Design review of the part built by this model. Coordinates are the model's own, in mm. Round coordinates to 2 decimals unless told otherwise and drop trailing zeros. Order: outer loops, then holes, each group sorted by start corner. A loop starts at its lowest first (then second) coordinate and runs counter-clockwise, first axis right, second up. Notation, with made-up numbers: M 14,-7 L 66,-7 A30 cw 66,32 Z; hole C 11,-9.75 d10. An arc over 180 degrees is marked long. Use a Markdown table: item, result. Add a question column.
(1) Take a section at B-B (x = -10). Write out the cut boundary in (y, z), then the cut area to 3 significant figures.
(2) To check wall thickness, follow probe 1 along Y at (x, z) = (10, 5); probe 2 along Y at (x, z) = (-27.5, 4.25); probe 3 along Y at (x, z) = (-32.5, 2.5). State the ranges of each line that lie inside material, in increasing order. Write a range as from..to.
(3) Take a section at D-D (y = 18.5). Write out the cut boundary in (x, z).
(4) Take a section at C-C (y = -10). Write out the cut boundary in (x, z).
(5) Take a section at A-A (z = 4.25). Write out the cut boundary in (x, y).
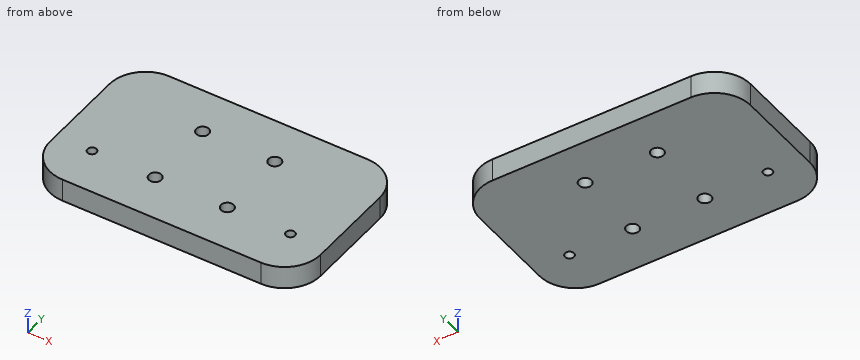
```python
from build123d import *

# Parameters (mm, degrees)
F0_W     = 75
F0_H     = 45
F0_R     = 1.25
F0_R_2   = 1.75
F1_DEPTH = 6.35
F2_R     = 10


with BuildPart() as f1:
    # F0 (on Top) → F1 (new body)
    with BuildSketch(Plane.XY):
        Rectangle(F0_W, F0_H)
        with Locations((-27.5, -10)):
            Circle(F0_R, mode=Mode.SUBTRACT)
        with Locations((-10, -10)):
            Circle(F0_R_2, mode=Mode.SUBTRACT)
        with Locations((10, -10)):
            Circle(F0_R_2, mode=Mode.SUBTRACT)
        with Locations((27.5, -10)):
            Circle(F0_R, mode=Mode.SUBTRACT)
        with Locations((-10, 10)):
            Circle(F0_R_2, mode=Mode.SUBTRACT)
        with Locations((10, 10)):
            Circle(F0_R_2, mode=Mode.SUBTRACT)
    extrude(amount=F1_DEPTH)

    # F2
    f2_edges = [f1.edges().sort_by_distance(p)[0] for p in [
        (-37.5, 22.5, 3.175),
        (37.5, 22.5, 3.175),
        (37.5, -22.5, 3.175),
        (-37.5, -22.5, 3.175),
    ]]
    fillet(f2_edges, radius=F2_R)


solid = f1.part
```
Verdict:
| question | item | result |
|---|---|---|
| 1 | outline | M -22.5,0 L -11.75,0 L -11.75,6.35 L -22.5,6.35 Z; M -8.25,0 L 8.25,0 L 8.25,6.35 L -8.25,6.35 Z; M 11.75,0 L 22.5,0 L 22.5,6.35 L 11.75,6.35 Z |
| 1 | area | 241 mm^2 |
| 2 | probe 1 | y = -22.5..-11.75, -8.25..8.25, 11.75..22.5 |
| 2 | probe 2 | y = -22.5..-11.25, -8.75..22.5 |
| 2 | probe 3 | y = -21.16..21.16 |
| 3 | outline | M -35.5,0 L 35.5,0 L 35.5,6.35 L -35.5,6.35 Z |
| 4 | outline | M -37.5,0 L -28.75,0 L -28.75,6.35 L -37.5,6.35 Z; M -26.25,0 L -11.75,0 L -11.75,6.35 L -26.25,6.35 Z; M -8.25,0 L 8.25,0 L 8.25,6.35 L -8.25,6.35 Z; M 11.75,0 L 26.25,0 L 26.25,6.35 L 11.75,6.35 Z; M 28.75,0 L 37.5,0 L 37.5,6.35 L 28.75,6.35 Z |
| 5 | outline | M -37.5,-12.5 A10 ccw -27.5,-22.5 L 27.5,-22.5 A10 ccw 37.5,-12.5 L 37.5,12.5 A10 ccw 27.5,22.5 L -27.5,22.5 A10 ccw -37.5,12.5 Z; hole C -27.5,-10 d2.5; hole C -10,-10 d3.5; hole C -10,10 d3.5; hole C 10,-10 d3.5; hole C 10,10 d3.5; hole C 27.5,-10 d2.5 |
